Could you check a few things on this model? Use its own coordinates, in mm. Face numbers are marked on the shaded views. A direction names the side the tool comes from. Round coordinates to 2 decimals unless told otherwise and drop trailing zeros. Loops run counter-clockwise (first coordinate to the right, second up) from the corner with the lowest first, then second, coordinate; pieces in that order, holes last. Notation, with made-up numbers: (44, 33) -> (56, 33) arc R18 cw to (56, 66) -> close; hole circle Ø8 at (33.25, -3.5). An arc over 180 degrees is marked (long way). Write each question's results on one line, items separated by ' | '.
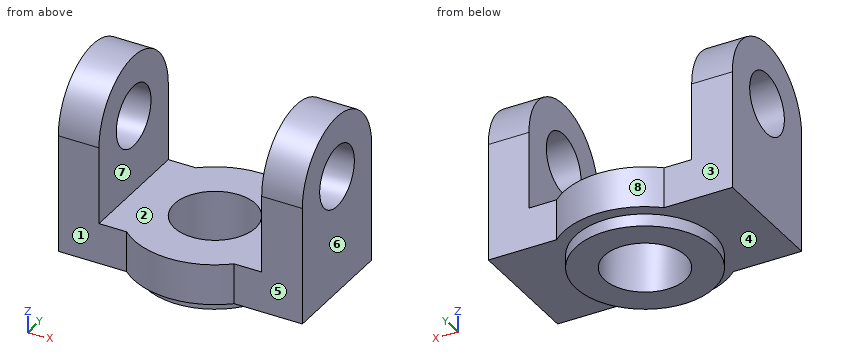
from build123d import *

# Parameters (mm, degrees)
F0_R     = 10
F1_DEPTH = 10
F4_R     = 17
F4_R_2   = 10
F5_DEPTH = 3
F3_R     = 7.5
F6_DEPTH = 10
F7_R     = 7.5
F8_DEPTH = 10


with BuildPart() as f1:
    # F0 (on Top) → F1 (new body)
    with BuildSketch(Plane.XY):
        with BuildLine():
            Line((-13.2287565553, 15), (-30, 15))
            Line((-30, 15), (-30, -15))
            Line((-30, -15), (-13.2287565553, -15))
            ThreePointArc((-13.2287565553, -15), (0, -20), (13.2287565553, -15))
            Line((13.2287565553, -15), (30, -15))
            Line((30, -15), (30, 15))
            Line((30, 15), (13.2287565553, 15))
            ThreePointArc((13.2287565553, 15), (0, 20), (-13.2287565553, 15))
        make_face()
        Circle(F0_R, mode=Mode.SUBTRACT)
    extrude(amount=F1_DEPTH)

    # F4 (on Top) → F5 (join)
    with BuildSketch(Plane.XY):
        Circle(F4_R)
        Circle(F4_R_2, mode=Mode.SUBTRACT)
    extrude(amount=-F5_DEPTH)

    # F3 (on offset) → F6 (join)
    with BuildSketch(Plane.YZ.offset(30)):
        with BuildLine():
            Line((-15, 29), (-15, 0))
            Line((-15, 0), (15, 0))
            Line((15, 0), (15, 29))
            ThreePointArc((15, 29), (0, 44), (-15, 29))
        make_face()
        with Locations((0, 29)):
            Circle(F3_R, mode=Mode.SUBTRACT)
    extrude(amount=-F6_DEPTH)

    # F7 (on face) → F8 (join)
    with BuildSketch(Plane(origin=(-30, 0, 0), x_dir=(0, -1, 0), z_dir=(-1, 0, 0))):
        with BuildLine():
            Line((-15, 29), (-15, 0))
            Line((-15, 0), (15, 0))
            Line((15, 0), (15, 29))
            ThreePointArc((15, 29), (0, 44), (-15, 29))
        make_face()
        with Locations((0, 29)):
            Circle(F7_R, mode=Mode.SUBTRACT)
    extrude(amount=-F8_DEPTH)


solid = f1.part
1) I need wall thicknesses on line 1 (Z direction, x = -24, y = 0); line 2 (Y direction, x = 0, z = 3); line 3 (X direction, y = 4, z = 18). Which ranges of each line are inside material? Lowest first, please.
Model answer:
line 1: z = 0 to 21.5, 36.5 to 44 | line 2: y = -20 to -10, 10 to 20 | line 3: x = -30 to -20, 20 to 30
2) I want a section at B-B, the plane y = 0. Write out the boundary of the cut face in (x, z), plus the area to 3 significant figures.
Model answer:
outline: (-30, 0) -> (-17, 0) -> (-17, -3) -> (-10, -3) -> (-10, 10) -> (-20, 10) -> (-20, 21.5) -> (-30, 21.5) -> close; (-30, 36.5) -> (-20, 36.5) -> (-20, 44) -> (-30, 44) -> close; (10, -3) -> (17, -3) -> (17, 0) -> (30, 0) -> (30, 21.5) -> (20, 21.5) -> (20, 10) -> (10, 10) -> close; (20, 36.5) -> (30, 36.5) -> (30, 44) -> (20, 44) -> close | area: 822 mm2
3) If we mould it in two halves opening along X, with no side actions, what happens to the marked faces 6, 7 and 8? For each: released by +X, released by -X, zero draft, split by the parting line, or undercut.
Model answer:
face 6: released by +X | face 7: undercut | face 8: split by the parting line
4) For the marked faces 1, 2, 3, 4 and 5, which set-ups out of +Z, -Z, +X, -X, +Y, -Y let a thin tool reach every point of the face, with its end or its side?
Model answer:
face 1: +Z, -Z, -X, -Y | face 2: +Z, +Y, -Y | face 3: +Z, -Z, -X, +Y | face 4: -Z | face 5: +Z, -Z, +X, -Y
5) I'm going to push flat-ended pins straight in: pin 1 (12 mm diameter, centred on x = 12.5, z = 2.5, fed in from -Y); pin 2 (5 mm diameter, centred on x = 23, z = 9, fed in from -Y); pin 3 (5 mm diameter, centred on x = -25, z = 19.5, fed in from +Y). Where does each tip first touch, or does it pass through?
Model answer:
pin 1: stops at y = -18.91 | pin 2: stops at y = -15 | pin 3: stops at y = 15
6) I want a section at C-C, the plane z = 17.5. Write out the boundary of the cut face in (x, y), plus the area to 3 significant figures.
Model answer:
outline: (-30, -15) -> (-20, -15) -> (-20, 15) -> (-30, 15) -> close; (20, -15) -> (30, -15) -> (30, 15) -> (20, 15) -> close | area: 600 mm2
7) I want a section at A-A, the plane x = 0. Write out the boundary of the cut face in (y, z).
Model answer:
outline: (-20, 0) -> (-17, 0) -> (-17, -3) -> (-10, -3) -> (-10, 10) -> (-20, 10) -> close; (10, -3) -> (17, -3) -> (17, 0) -> (20, 0) -> (20, 10) -> (10, 10) -> close
8) I want a section at D-D, the plane z = 1. Write out the boundary of the cut face in (x, y).
Model answer:
outline: (-30, -15) -> (-13.23, -15) arc R20 ccw to (13.23, -15) -> (30, -15) -> (30, 15) -> (13.23, 15) arc R20 ccw to (-13.23, 15) -> (-30, 15) -> close; hole circle Ø20 at (0, 0)
